For this review, take the finished solid that the model builds, in its own axes (mm). Face numbers are marked on the shaded views. A direction names the side the tool comes from. Coordinates: 2 decimals unless noted, no trailing zeros. Write each loop counter-clockwise with the first axis right and the second up, starting at its lowest first coordinate (ties: lowest second). Pieces come first, ordered by that corner, then holes. Notation, with made-up numbers: (26.5, -8) - (73.5, -8) arc R20 ccw to (73.5, 17) - close; hole circle Ø1 at (28, 33.5). An arc over 180 degrees is marked (long way). Use one line per item in the form item = value. Start each with the question number.
1) We need section D-D (x = -2.75). Give the boundary of the cut face in (y, z), plus the area to 3 significant figures.
2) We need section B-B (z = 12). Give the boundary of the cut face in (x, y) (3 decimals), plus the area to 3 significant figures.
3) Insertion check: P1, Ø3, axis at x = 3.5, z = 3.5, coming from the +Y side; P2, Ø1, axis at x = 2.5, y = -0.5, coming from the -Z side; P3, Ø5, axis at x = -4.5, z = 2, coming from the -Y side; P4, Ø6, axis at x = 0.5, z = 7, coming from the +Y side (3 decimals). Each pin has a flat end and moves straight along its axis. Give the tip position at first contact, or say it passes through.
4) Tool access review of the marked faces 4, 5 and 6: name each direction out of +Z, -Z, +X, -X, +Y, -Y from which nothing blocks a thin tool from reaching the whole face with its end or side.
5) We need section A-A (y = 0). Give the boundary of the cut face in (x, z) (3 decimals).
6) For L1, parallel to Z at x = 4.25, y = -4.25; L2, parallel to X at y = 0.25, z = 2.25; L3, parallel to Y at x = 1.25, z = 7.75, list the stretches that pass through material, from the lowest coordinate up. Write a range as from..to.
7) We need section C-C (x = 0). Give the boundary of the cut face in (y, z) (3 decimals).
8) Mouldability with a two-part tool opening along X and no side actions: class the marked faces 1, 2 and 3 as pulls with the +X half, pulls with the -X half, needs draft (parallel to the pull), parting line crosses it, or undercut.
```python
from build123d import *

# Parameters (mm, degrees)
F0_R     = 3.125
F1_DEPTH = 14
F0_R_2   = 6.5
F2_DEPTH = 1
F4_DEPTH = 4.5


with BuildPart() as f1:
    # F0 (on Top) → F1 (new body)
    with BuildSketch(Plane.XY):
        Circle(F0_R)
    extrude(amount=F1_DEPTH)

    # F0 (on Top) → F2 (join)
    with BuildSketch(Plane.XY):
        Circle(F0_R_2)
        Circle(F0_R, mode=Mode.SUBTRACT)
    extrude(amount=F2_DEPTH)

    # F3 (on face) → F4 (cut)
    with BuildSketch(Plane.XY.offset(14)):
        with BuildLine():
            Line((0.625, -3.0618621785), (0.625, 3.0618621785))
            ThreePointArc((0.625, 3.0618621785), (0, 3.125), (-0.625, 3.0618621785))
            Line((-0.625, 3.0618621785), (-0.625, -3.0618621785))
            ThreePointArc((-0.625, -3.0618621785), (0, -3.125), (0.625, -3.0618621785))
        make_face()
    extrude(amount=-F4_DEPTH, mode=Mode.SUBTRACT)


solid = f1.part
```
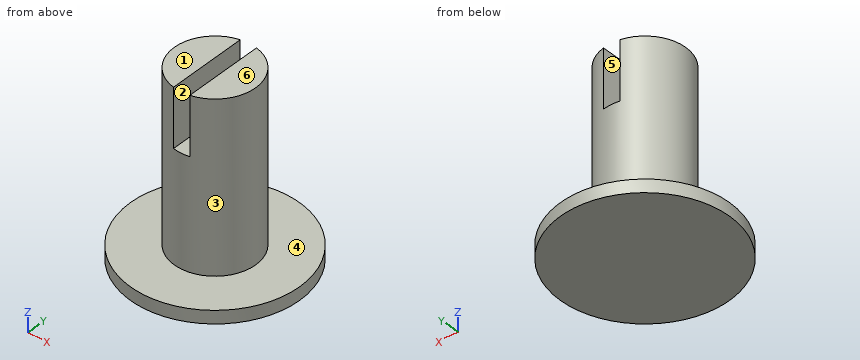
Determined:
q1.outline = (-5.89, 0) - (5.89, 0) - (5.89, 1) - (1.48, 1) - (1.48, 14) - (-1.48, 14) - (-1.48, 1) - (-5.89, 1) - close
q1.area = 50.4 mm²
q2.outline = (-0.625, -3.062) - (-0.625, 3.062) arc R3.125 ccw to start; (0.625, -3.062) arc R3.125 ccw to (0.625, 3.062) - close
q2.area = 22.9 mm²
q3.P1 = 2.4
q3.P2 = 0
q3.P3 = -6.11
q3.P4 = 3.125
q4.face_4 = +Z
q4.face_5 = +Z, +Y, -Y
q4.face_6 = +Z, +X, -X, +Y, -Y
q5.outline = (-6.5, 0) - (6.5, 0) - (6.5, 1) - (3.125, 1) - (3.125, 14) - (0.625, 14) - (0.625, 9.5) - (-0.625, 9.5) - (-0.625, 14) - (-3.125, 14) - (-3.125, 1) - (-6.5, 1) - close
q6.L1 = 0..1
q6.L2 = -3.11..3.11
q6.L3 = -2.86..2.86
q7.outline = (-6.5, 0) - (6.5, 0) - (6.5, 1) - (3.125, 1) - (3.125, 9.5) - (-3.125, 9.5) - (-3.125, 1) - (-6.5, 1) - close
q8.face_1 = needs draft
q8.face_2 = undercut
q8.face_3 = parting line crosses it
